from build123d import *

# Parameters (mm, degrees)
SKETCH1_W               = 38.1
SKETCH1_H               = 25.4
SKETCH1_W_2             = 31.75
SKETCH1_H_2             = 19.05
BOSS_EXTRUDE1_DEPTH     = 169.106596
CUT_EXTRUDE1_DEPTH      = 174.810071085
CUT_EXTRUDE1_DEPTH_BACK = 174.810071085
SKETCH2_R               = 2.413
FILLET7_R               = 12.7


with BuildPart() as part:
    # Sketch1 → Boss-Extrude1 (new body)
    with BuildSketch(Plane(origin=(0, 0, 0), x_dir=(1, 0, 0), z_dir=(0, 1, 0))):
        Rectangle(SKETCH1_W, SKETCH1_H)
        Rectangle(SKETCH1_W_2, SKETCH1_H_2, mode=Mode.SUBTRACT)
    extrude(amount=BOSS_EXTRUDE1_DEPTH)

    # Sketch2 → Cut-Extrude1 (cut, two sides: drawn at the far end of the back side and taken through both)
    with BuildSketch(Plane(origin=(19.05, 0, 0), x_dir=(0, 0, -1), z_dir=(1, 0, 0)).offset(-CUT_EXTRUDE1_DEPTH_BACK)):
        with Locations((0, 156.406596)):
            Circle(SKETCH2_R)
        with Locations((0, 12.7)):
            Circle(SKETCH2_R)
    extrude(amount=CUT_EXTRUDE1_DEPTH + CUT_EXTRUDE1_DEPTH_BACK, mode=Mode.SUBTRACT)

    # Fillet7
    # the kernel refuses this fillet: 12.7 mm, written as the material it takes off along each edge
    with BuildSketch(Plane(origin=(50.8, 169.106596, -12.7), x_dir=(0, 0, 1), z_dir=(-1, 0, 0)), Plane(origin=(-50.8, 0, 12.7), x_dir=(0, 1, 0), z_dir=(1, 0, 0))) as fillet7_piece_1:
        with BuildLine():
            CenterArc((FILLET7_R, -FILLET7_R), FILLET7_R, 90, 90)
            Line((0, -FILLET7_R), (0, 0))
            Line((0, 0), (FILLET7_R, 0))
        make_face()
    extrude(amount=101.6, mode=Mode.SUBTRACT)
    with BuildSketch(Plane(origin=(50.8, 0, -12.7), x_dir=(0, 0, 1), z_dir=(-1, 0, 0)), Plane(origin=(-50.8, 169.106596, 12.7), x_dir=(0, -1, 0), z_dir=(1, 0, 0))) as fillet7_piece_2:
        with BuildLine():
            CenterArc((FILLET7_R, FILLET7_R), FILLET7_R, 180, 90)
            Line((0, FILLET7_R), (0, 0))
            Line((0, 0), (FILLET7_R, 0))
        make_face()
    extrude(amount=101.6, mode=Mode.SUBTRACT)


solid = part.part
Design review of the part built by this model. Coordinates are the model's own, in mm. A direction names the side the tool comes from. Coordinates: 2 decimals unless noted, no trailing zeros. Order: outer loops, then holes, each group sorted by start corner. A loop starts at its lowest first (then second) coordinate and runs counter-clockwise, first axis right, second up. Notation, with made-up numbers: M 35,83 L 45,83 A26 cw 45,115 Z; hole C 49.25,32 d3. An arc over 180 degrees is marked long. Use a Markdown table: item, result.
(1) Wall thickness on probe 1 along Y at (x, z) = (-18.4, 0); probe 2 along Z at (x, y) = (18.1, 12.7); probe 3 along Z at (x, y) = (-5.5, 24) (3 decimals): over which ranges is each line inside the solid? List them lowest first.
Worked answers:
| item | result |
|---|---|
| probe 1 | y = 0 to 10.29, 15.11 to 153.99, 158.82 to 169.11 |
| probe 2 | z = -12.7 to -2.41, 2.41 to 12.7 |
| probe 3 | z = -12.7 to -9.525, 9.525 to 12.7 |
(2) Add section C-C (z = -7.25). Give the boundary of the cut face in (x, y) (3 decimals), then the cut area to 3 significant figures.
Worked answers:
| item | result |
|---|---|
| outline | M -19.05,2.273 L -15.875,2.273 L -15.875,166.834 L -19.05,166.834 Z; M 15.875,2.273 L 19.05,2.273 L 19.05,166.834 L 15.875,166.834 Z |
| area | 1,040 mm2 |
(3) For faces 1 (the cylindrical face through (0.267, 6.11, 10.856)), 2 (the flat face through (-15.875, 83, 0)), list the 3-axis set-ups (+Z, -Z, +X, -X, +Y, -Y) from which the entire face can be reached by the end or side of a thin tool; tool diameter is ignored.
Worked answers:
| item | result |
|---|---|
| face 1 | +X, -X, -Y |
| face 2 | +Y, -Y |
(4) Add section A-A (y = 90). Give the boundary of the cut face in (x, z) (3 decimals), then the cut area to 3 significant figures.
Worked answers:
| item | result |
|---|---|
| outline | M -19.05,-12.7 L 19.05,-12.7 L 19.05,12.7 L -19.05,12.7 Z; hole M -15.875,-9.525 L 15.875,-9.525 L 15.875,9.525 L -15.875,9.525 Z |
| area | 363 mm2 |
(5) Add section B-B (x = -8.5). Give the boundary of the cut face in (y, z) (3 decimals), then the cut area to 3 significant figures.
Worked answers:
| item | result |
|---|---|
| outline | M 4.3,-9.525 A12.7 ccw 12.7,-12.7 L 156.407,-12.7 A12.7 ccw 164.807,-9.525 Z; M 4.3,9.525 L 164.807,9.525 A12.7 ccw 156.407,12.7 L 12.7,12.7 A12.7 ccw Z |
| area | 986 mm2 |
(6) Draft analysis for pull direction X (two halves, no side actions). For faces 3 (the cylindrical face through (17.44, 10.344, 0.523)), 4 (the flat face through (-19.05, 83, 0)), 5 (the flat face through (0, 83, -9.525)), state which applies: released by +X, released by -X, zero draft, split by the parting line, or undercut.
Worked answers:
| item | result |
|---|---|
| face 3 | zero draft |
| face 4 | released by -X |
| face 5 | undercut |
